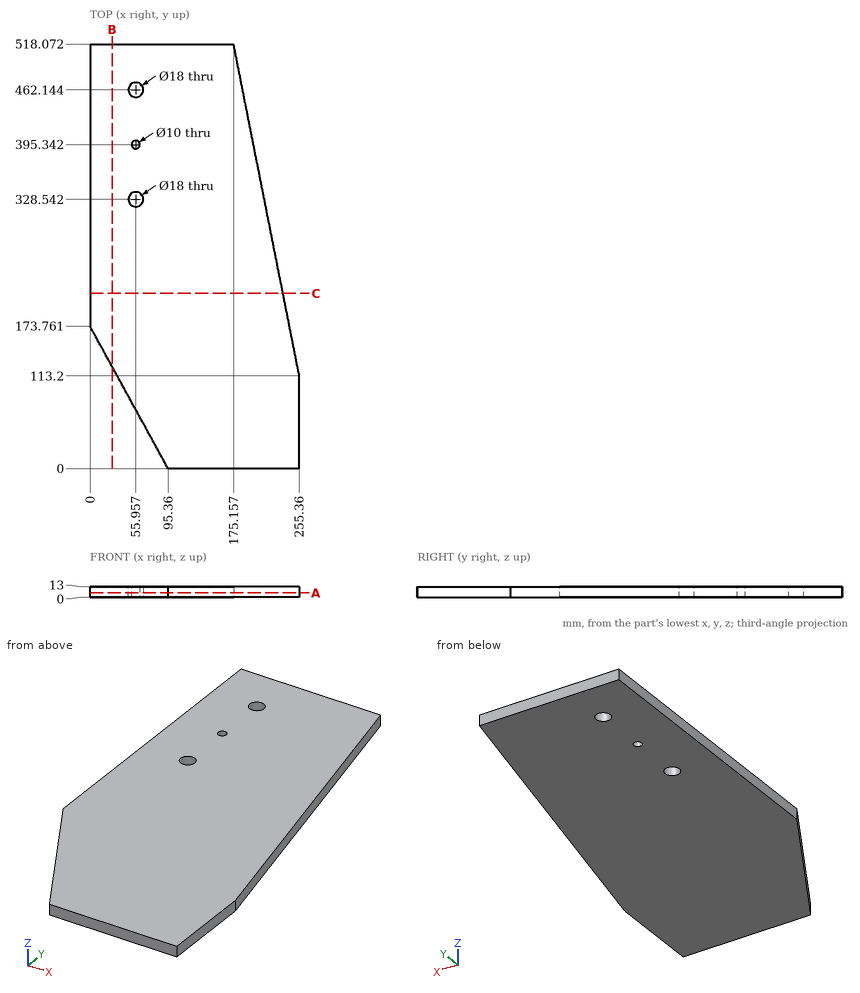
Verification items for this drawing (mm, ordinates from the low corner). Round coordinates to 2 decimals unless told otherwise and drop trailing zeros. Order: outer loops, then holes, each group sorted by start corner. A loop starts at its lowest first (then second) coordinate and runs counter-clockwise, first axis right, second up. Notation, with made-up numbers: (49.5, -17) - (76.5, -17) arc R25 cw to (76.5, 12) - close; hole circle Ø1 at (4, 89). An arc over 180 degrees is marked (long way). Use CSV: the item, a comma, the result in double quotes. Start each with the question number.
1) Section check C-C, the plane y = 214. Record the cut outline in (x, z).
2) Thickness scan on L1, parallel to X at y = 267, z = 9.75; L2, parallel to X at y = 330, z = 12 (1 decimal); L3, parallel to X at y = 364.5, z = 10.75. Record the ranges inside material, lowest first.
3) Section check A-A, the plane z = 5.5. Record the cut outline in (x, y).
4) Go/stop test with a flat-tipped pin: P1, Ø6, axis at y = 274, z = 3, coming from the -X side. Record where the tip stops, or that it passes through.
5) Section check B-B, the plane x = 27. Record the cut outline in (y, z).
Answers:
1,outline,"(0, 0) - (235.39, 0) - (235.39, 13) - (0, 13) - close"
2,L1,"x = 0 to 224.89"
2,L2,"x = 0 to 47.1, 64.8 to 212.4"
2,L3,"x = 0 to 205.58"
3,outline,"(0, 173.76) - (95.36, 0) - (255.36, 0) - (255.36, 113.2) - (175.16, 518.07) - (0, 518.07) - close; hole circle Ø18 at (55.96, 328.54); hole circle Ø18 at (55.96, 462.14); hole circle Ø10 at (55.96, 395.34)"
4,P1,"stops at x = 0"
5,outline,"(124.56, 0) - (518.07, 0) - (518.07, 13) - (124.56, 13) - close"
